Geometry check sheet. Reference: the model listing, model coordinates, mm. A direction names the side the tool comes from. Round coordinates to 2 decimals unless told otherwise and drop trailing zeros. Write each loop counter-clockwise with the first axis right and the second up, starting at its lowest first coordinate (ties: lowest second). Pieces come first, ordered by that corner, then holes.
Item 1: Draft check along Z on faces 4 (the face through (-8, 2, 6.35)), 5 (the face through (-8, 2, 0)), 6 (the face through (-0.12, 19.05, 3.13)). Enter one of: pulls with the +Z half, pulls with the -Z half, needs draft (parallel to the pull), parting line crosses it, or undercut.
Item 2: Cross-section at D-D (x = -22). Enter the section's corners in (y, z).
Item 3: Scan lines: probe 1 along X at (y, z) = (-5.5, 1.5); probe 2 along X at (y, z) = (-54, 4). Record each from-to range of solid material in increasing order.
Item 4: Cross-section at B-B (z = 4.75). State how many separate pieces and enclosed holes the cut face has, then the cut area to 3 significant figures.
Item 5: Access from +Z, -Z, +X, -X, +Y, -Y to the whole of each face (thin tool, end or side, straight path). Record for faces 1 (the face through (11.368, -71.045, 3.131)), 2 (the face through (4.666, -32.098, 3.131)), 3 (the face through (-11.368, -71.045, 3.131)).
Item 6: Depth check by flat-ended pin: P1, Ø1, axis at y = -15, z = 1, coming from the +X side. Enter the tip coordinate at first touch or a pass-through.
Item 7: Cross-section at A-A (y = 0). Enter the section's corners in (x, z).
Item 8: Cross-section at C-C (y = 12.7). Enter the section's corners in (x, z).
Autodesk Inventor part; units mm, degrees
ref_plane "YZ Plane" through (0, 0, 0) normal (1, 0, 0) x (0, 1, 0)
ref_plane "XZ Plane" through (0, 0, 0) normal (0, 1, 0) x (-1, 0, 0)
ref_plane "XY Plane" through (0, 0, 0) normal (0, 0, 1) x (1, 0, 0)
sketch "Sketch1" plane through (0, 0, 0) normal (0, 0, 1) x (1, 0, 0)
  circle A0 centre (0, 0) radius 7.1437
  line L0 (0, 0) -> (0, 12.7) construction
  circle A1 centre (0, 12.7) radius 1.7526
  circle A2 centre (-10.9985, 6.35) radius 1.7526
  circle A3 centre (-10.9985, -6.35) radius 1.7526
  circle A4 centre (0, -12.7) radius 1.7526
  circle A5 centre (10.9985, -6.35) radius 1.7526
  circle A6 centre (10.9985, 6.35) radius 1.7526
  circle A7 centre (0, 0) radius 19.05
  circle A8 centre (0, 0) radius 76.2 construction
  line L1 (0, 0) -> (-13.232, -75.0424) construction
  line L2 (-13.232, -75.0424) -> (4.8119, -36.3472) construction
  line L3 (-13.232, -75.0424) -> (-9.0429, -66.0589)
  line L4 (-9.0429, -66.0589) -> (-18.8254, -2.9166)
  circle A9 centre (0, 0) radius 66.675 construction
  line L5 (0, 0) -> (0, -76.2) construction
  arc A10 (-13.232, -75.0424) -> (0, -76.2) centre (0, 0) ccw
  line L6 (13.232, -75.0424) -> (9.0429, -66.0589)
  line L7 (9.0429, -66.0589) -> (18.8254, -2.9166)
  arc A11 (0, -76.2) -> (13.232, -75.0424) centre (0, 0) ccw
  arc A12 (-2.5837, -18.874) -> (-6.1519, -22.5057) centre (-3.0143, -22.0196) ccw
  line L8 (-6.1519, -22.5057) -> (-3.1376, -41.9621)
  arc A13 (-3.1376, -41.9621) -> (0, -44.651) centre (0, -41.476) ccw
  arc A14 (6.1519, -22.5057) -> (2.5837, -18.874) centre (3.0143, -22.0196) ccw
  line L9 (6.1519, -22.5057) -> (3.1376, -41.9621)
  arc A15 (0, -44.651) -> (3.1376, -41.9621) centre (0, -41.476) ccw
  circle A16 centre (0, 0) radius 50.8 construction
  line L10 (-32.6536, 38.9151) -> (-18.1201, -5.8791)
  line L11 (-32.6536, 38.9151) -> (0, 0) construction
  arc A17 (0, 50.8) -> (-32.6536, 38.9151) centre (0, 0) ccw
  line L12 (32.6536, 38.9151) -> (18.1201, -5.8791)
  line L13 (32.6536, 38.9151) -> (0, 0) construction
  arc A18 (32.6536, 38.9151) -> (0, 50.8) centre (0, 0) ccw
  arc A19 (9.3927, 20.1427) -> (-9.3927, 20.1427) centre (0, 0) ccw construction
  arc A20 (10.7345, 23.0202) -> (-10.7345, 23.0202) centre (0, 0) ccw
  arc A21 (8.0509, 17.2652) -> (-8.0509, 17.2652) centre (0, 0) ccw
  arc A22 (8.0509, 17.2652) -> (10.7345, 23.0202) centre (9.3927, 20.1427) ccw
  arc A23 (-10.7345, 23.0202) -> (-8.0509, 17.2652) centre (-9.3927, 20.1427) ccw
  line L14 (-9.3927, 20.1427) -> (0, 0) construction
  line L15 (0, 0) -> (9.3927, 20.1427) construction
  line L16 (0, -72.9607) -> (-1.5036, -76.1852)
  line L17 (-1.5036, -76.1852) -> (0, -72.9607)
  line L18 (1.5036, -76.1852) -> (0, -72.9607)
  point P0 (-18.5915, -4.4261)
  point P1 (18.5915, -4.4261)
  point P2 (2.5837, -18.874)
  point P3 (-11.1375, -70.5506)
  point P4 (8.0509, 17.2652)
  point P5 (-8.0509, 17.2652)
  dimension "d10" = 133.35
  dimension "d0" = 14.2875
  dimension "d1" = 12.7
  dimension "d2" = 3.5052
  dimension "d5" = 360
  dimension "d7" = 38.1
  dimension "d8" = 152.4
  dimension "d9" = 15
  dimension "d11" = 10
  dimension "d12" = 6.35
  dimension "d14" = 6.35
  dimension "d15" = 9.525
  dimension "d16" = 101.6
  dimension "d17" = 80
  dimension "d18" = 50
  dimension "d19" = 3.175
  dimension "d20" = 22.225
  dimension "d25" = 11.1125
extrude "Extrusion1" add sketch "Sketch1" along normal blind 6.35 contours A7 | A7 A22 A20 A23 L4 L10 A17 A18 L12 L7 | L7 L12 A7 | L12 L7 L6 A11 L18 L16 A10 L3 L4 L10 A7 A12 L8 A13 A15 L9 A14 | A7 L10 L4
fillet "Fillet1" radius 3.175 5 edges at (18.5915, -4.4261, 3.175) (9.0429, -66.0589, 3.175) (-18.5915, -4.4261, 3.175) (-9.0429, -66.0589, 3.175) (0, -72.9607, 3.175)
sketch "Sketch2" plane through (0, 0, 6.35) normal (0, 0, 1) x (1, 0, 0)
  arc A0 (1.5036, -76.1852) -> (13.232, -75.0424) centre (0, 0) ccw
  circle A1 centre (0, 0) radius 76.2 construction
properties part number "Blade (Bar 3)" material "Steel, Alloy"
Resolved:
1. face 4: pulls with the +Z half
1. face 5: pulls with the -Z half
1. face 6: needs draft
2. outline: (6.08, 0) - (45.79, 0) - (45.79, 6.35) - (6.08, 6.35) - close
3. probe 1: x = -18.43 to -12.53, -9.47 to -4.56, 4.56 to 9.47, 12.53 to 18.43
3. probe 2: x = -10.91 to 10.91
4. separate pieces: 1
4. enclosed holes: 9
4. area: 4,070 mm2
5. face 1: +Z, -Z, +X
5. face 2: +Z, -Z
5. face 3: +Z, -Z, -X
6. P1: stops at x = 17.03
7. outline: (-20.03, 0) - (-7.14, 0) - (-7.14, 6.35) - (-20.03, 6.35) - close; (7.14, 0) - (20.03, 0) - (20.03, 6.35) - (7.14, 6.35) - close
8. outline: (-24.15, 0) - (-1.75, 0) - (-1.75, 6.35) - (-24.15, 6.35) - close; (1.75, 0) - (24.15, 0) - (24.15, 6.35) - (1.75, 6.35) - close
